from build123d import *

# Parameters (mm, degrees)
R_VOLUTION1_ANGLE            = 20
ESQUISSE4_R                  = 1.25
ENL_V_MAT_EXTRU_1_DEPTH      = 10
ESQUISSE7_R                  = 1.25
ENL_V_MAT_EXTRU_2_DEPTH      = 10
R_P_TITION_CIRCULAIRE1_COUNT = 2
R_P_TITION_CIRCULAIRE1_ANGLE = 10
R_VOLUTION2_ANGLE            = 1
R_VOLUTION2_OTHER_WAY_ANGLE  = 1


with BuildPart() as part:
    # Esquisse2 → Révolution1 (revolve)
    with BuildSketch(Plane.XY):
        Polygon((0, 0), (20, 0), (20, 5), (5, 5), (5, 20), (0, 20), align=None)
    revolve(axis=Axis((84, 0, 0), (0, 1, 0)), revolution_arc=R_VOLUTION1_ANGLE)

    # Esquisse4 → Enlèv. mat.-Extru.1 (cut)
    with BuildSketch(Plane(origin=(0, 5, 0), x_dir=(1, 0, 0), z_dir=(0, 1, 0))):
        with Locations(Location((14.93630342, -18.505561725, 0), (0, 0, 270))):
            Circle(ESQUISSE4_R)
        with Locations(Location((12.772079086, -6.231635606, 0), (0, 0, 270))):
            Circle(ESQUISSE4_R)
    extrude(amount=-ENL_V_MAT_EXTRU_1_DEPTH, mode=Mode.SUBTRACT)

    # Esquisse7 → Enlèv. mat.-Extru.2 (cut)
    with BuildSketch(Plane(origin=(-0.318429013, 0, 0.027858929), x_dir=(0, -1, 0), z_dir=(-0.9961946980917459, 0, 0.08715574274765504))):
        with Locations(Location((-12.5, 7.321082391, 0), (0, 0, 90))):
            Circle(ESQUISSE7_R)
    enl_v_mat_extru_2 = extrude(amount=-ENL_V_MAT_EXTRU_2_DEPTH, mode=Mode.SUBTRACT)

    # Répétition circulaire1: Enlèv. mat.-Extru.2 ×2 about axis
    r_p_tition_circulaire1_axis = Axis((84, 0, 0), (0, 1, 0))
    for i in range(1, R_P_TITION_CIRCULAIRE1_COUNT):
        add(enl_v_mat_extru_2.rotate(r_p_tition_circulaire1_axis, i * R_P_TITION_CIRCULAIRE1_ANGLE / (R_P_TITION_CIRCULAIRE1_COUNT - 1)), mode=Mode.SUBTRACT)

    # Esquisse9 → Révolution2 (revolve)
    with BuildSketch(Plane(origin=(2.532909927, 0, 14.36484602), x_dir=(-0.9848077530122081, 0, 0.17364817766693072), z_dir=(-0.17364817766693072, 0, -0.9848077530122081))):
        Polygon((-3.746639624, 5), (-3.746639624, 20), (-18.746639624, 5), align=None)
    revolve(axis=Axis((84, 0, 0), (0, -1, 0)), revolution_arc=R_VOLUTION2_ANGLE)

    # Esquisse9 → Révolution2 other way (revolve)
    with BuildSketch(Plane(origin=(2.532909927, 0, 14.36484602), x_dir=(-0.9848077530122081, 0, 0.17364817766693072), z_dir=(-0.17364817766693072, 0, -0.9848077530122081))):
        Polygon((-3.746639624, 5), (-3.746639624, 20), (-18.746639624, 5), align=None)
    revolve(axis=Axis((84, 0, 0), (0, 1, 0)), revolution_arc=R_VOLUTION2_OTHER_WAY_ANGLE)


solid = part.part
Work out the finished part from the listing and answer in its coordinate system (mm). A direction names the side the tool comes from. Round coordinates to 2 decimals unless told otherwise and drop trailing zeros. Write each loop counter-clockwise with the first axis right and the second up, starting at its lowest first coordinate (ties: lowest second). Pieces come first, ordered by that corner, then holes.
1) A tool of negligible diameter and unlimited length cuts with its end or side. For faces 4 (the flat face through (10.667, 9.272, 14.254)), 5 (the flat face through (12, 0, 11)), 6 (the flat face through (10.214, 9.272, 11.687)), from which of +Z, -Z, +X, -X, +Y, -Y can it reach the whole face along a straight path? Write none if from no direction.
2) The mould has two halves that part along Z. Classify faces 1 (the flat face through (10.15, 3.47, 26.88)), 2 (the cylindrical face through (20.945, 2.535, 10.959)), 3 (the cylindrical face through (15.99, 2.54, 19.18)): pulls with the +Z half, pulls with the -Z half, needs draft (parallel to the pull), parting line crosses it, or undercut.
3) Straight lines are drawn through the part: line 1 (Y direction, x = 8, z = 16); line 2 (X direction, y = 2.25, z = 19.5); line 3 (X direction, y = 2.5, z = 10). For each, find the intervals that lie inside material, in ascending order.
4) A cutting plane is placed at A-A (y = 8.25). Give the vertices of the cut face in (x, z), plus the area to 3 significant figures.
5) Given pin 1 Ø5 at (y, z) = (15, 5.5) entering from +X; pin 2 Ø10 at (x, z) = (16.5, 23) entering from +Y; pin 3 Ø5 at (x, y) = (9.5, 15.5) entering from -Z, each flat-ended and moving along its own axis, determine where each tip first touches the part or whether it passes through.
6) A cutting plane is placed at D-D (y = 17.25). Give the vertices of the cut face in (x, z).
7) A cutting plane is placed at C-C (y = 13). Give the vertices of the cut face in (x, z), plus the area to 3 significant figures.
8) A cutting plane is placed at B-B (z = 18.25). Give the vertices of the cut face in (x, y).
Completed:
1. face 4: +X, +Y
1. face 5: +Z, -Z, +X, -X, -Y
1. face 6: -Z, +Y
2. face 1: pulls with the +Z half
2. face 2: pulls with the -Z half
2. face 3: undercut
3. line 1: y = 0 to 5
3. line 2: x = 2.29 to 14.18, 15.69 to 23.04
3. line 3: x = 0.6 to 20.79
4. outline: (0, 0) - (5, 0) arc R79 cw to (9.76, 27.02) - (5.07, 28.73) arc R84 ccw to start; (6, 12.35) - (17.6, 10.52) arc R67.23 cw to (18.01, 12.83) - (6.47, 15.07) arc R78.98 ccw to start
4. area: 172 mm2
5. pin 1: stops at x = 5.41
5. pin 2: stops at y = 5
5. pin 3: stops at z = 11.46
6. outline: (0, 0) - (5, 0) arc R79 cw to (9.76, 27.02) - (5.07, 28.73) arc R84 ccw to start; (6, 12.35) - (8.71, 11.92) arc R76.23 cw to (9.17, 14.54) - (6.47, 15.07) arc R78.98 ccw to start
7. outline: (0, 0) - (5, 0) arc R79 cw to (5.21, 5.74) - (0.23, 6.18) arc R84 ccw to start; (0.43, 8.46) - (5.41, 8.03) arc R79 cw to (7.4, 19.34) - (2.57, 20.63) arc R84 ccw to start; (3.17, 22.85) - (8, 21.55) arc R79 cw to (9.76, 27.02) - (5.07, 28.73) arc R84 ccw to start; (6, 12.35) - (12.91, 11.26) arc R71.98 cw to (13.35, 13.73) - (6.47, 15.07) arc R78.98 ccw to start
7. area: 138 mm2
8. outline: (2.01, 0) - (13.71, 0) - (13.71, 5) - (7.14, 5) - (7.14, 20) - (2.01, 20) - close; (16.16, 0) - (22.66, 0) - (22.66, 5) - (16.16, 5) - close
